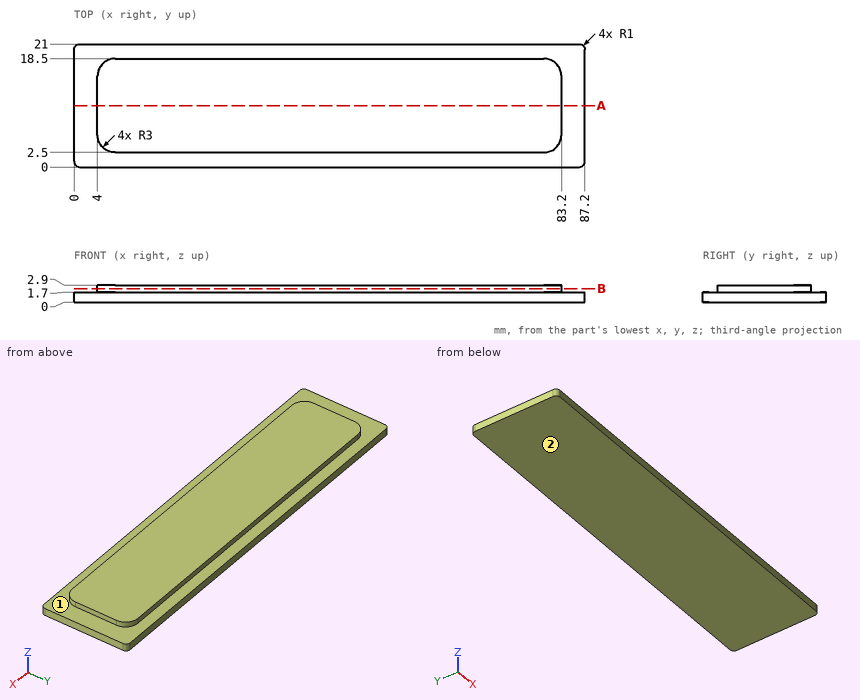
Print and shaded views of the part. All mm, measured from the part's lowest x, y and z. Coordinates: 2 decimals unless noted, no trailing zeros. Loops run counter-clockwise (first coordinate to the right, second up) from the corner with the lowest first, then second, coordinate; pieces in that order, holes last. Notation, with made-up numbers: (22.5, 12) -> (52.5, 12) arc R26 ccw to (52.5, 31) -> close; hole circle Ø2 at (-38.5, 73). An arc over 180 degrees is marked (long way). Use one line per item in the form item = value. Start each with the question number.
(1) Probe probe 1 along X at (y, z) = (15, 2.65); probe 2 along Y at (x, z) = (73, 1.95); probe 3 along Z at (x, y) = (52.5, 1.5). List the from-to ranges inside material, lowest first. Write a range as from..to.
(2) Pull direction Z, two halves, no side cores. Call the marked faces 1 and 2: pulls with the +Z half, pulls with the -Z half, needs draft (parallel to the pull), parting line crosses it, or undercut.
(3) Cut at B-B on z = 2.3. Give the cut face in (x, y).
(4) Cut at A-A on y = 10.5. Give the cut face in (x, z), and give its area (3 significant figures).
Values:
q1.probe_1 = 4..83.2
q1.probe_2 = 2.5..18.5
q1.probe_3 = 0..1.7
q2.face_1 = pulls with the +Z half
q2.face_2 = pulls with the -Z half
q3.outline = (4, 5.5) arc R3 ccw to (7, 2.5) -> (80.2, 2.5) arc R3 ccw to (83.2, 5.5) -> (83.2, 15.5) arc R3 ccw to (80.2, 18.5) -> (7, 18.5) arc R3 ccw to (4, 15.5) -> close
q4.outline = (0, 0) -> (87.2, 0) -> (87.2, 1.7) -> (83.2, 1.7) -> (83.2, 2.9) -> (4, 2.9) -> (4, 1.7) -> (0, 1.7) -> close
q4.area = 243 mm2
